For this review, use the dimensioned drawing (mm, ordinates from the lowest corner) and the shaded views. A direction names the side the tool comes from. Give positions to 0.01 mm unless a question says otherwise; leave off trailing zeros. Order: outer loops, then holes, each group sorted by start corner. A loop starts at its lowest first (then second) coordinate and runs counter-clockwise, first axis right, second up. Notation, with made-up numbers: M 57,-3 L 93,-3 A24 cw 93,26 Z; hole C 79.25,-17.5 d11. An arc over 180 degrees is marked long. Answer as CSV lines item,"result". Start each with the question number.
1. We need section A-A, the plane x = 6. Give the boundary of the cut face in (y, z), and give its area (3 significant figures).
2. We need section C-C, the plane z = 6. Give the boundary of the cut face in (x, y), and give its area (3 significant figures).
3. We need section B-B, the plane y = 3. Give the boundary of the cut face in (x, z), and give its area (3 significant figures).
4. We need section D-D, the plane y = 17.25. Give the boundary of the cut face in (x, z), and give its area (3 significant figures).
5. Clearance check with a flat-ended pin moving along its axis: P1, Ø5, axis at y = 18, z = 4.5, coming from the +X side. State where the tip first meets the part, or that it passes through.
6. For line 1 along X through (y, z) = (6, 6); line 2 along Y through (x, z) = (7.5, 3.5); line 3 along Y through (x, z) = (1.75, 3.5), list the stretches that pass through material, from the lowest coordinate up.
7. Mouldability with a two-part tool opening along X and no side actions: class the marked faces 3, 4 and 5 as pulls with the +X half, pulls with the -X half, needs draft (parallel to the pull), parting line crosses it, or undercut.
8. Machinability: for the marked faces 1 and 2, which of the approach directions +Z, -Z, +X, -X, +Y, -Y give a long, thin tool a straight path to every point of the face, cutting with its end or side? Answer none if there is none.
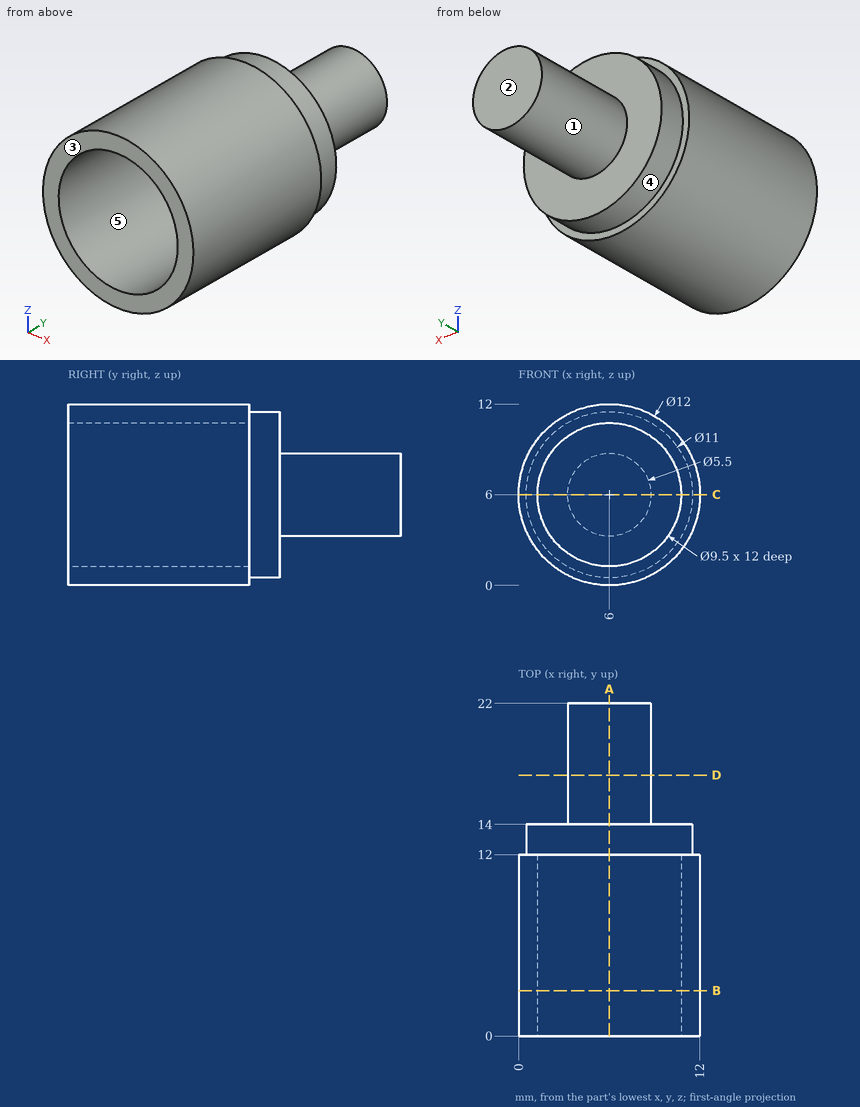
Result set:
1,outline,"M 0,0 L 12,0 L 12,0.5 L 14,0.5 L 14,3.25 L 22,3.25 L 22,8.75 L 14,8.75 L 14,11.5 L 12,11.5 L 12,12 L 0,12 L 0,10.75 L 12,10.75 L 12,1.25 L 0,1.25 Z"
1,area,"96.0 mm2"
2,outline,"M 0,0 L 1.25,0 L 1.25,12 L 10.75,12 L 10.75,0 L 12,0 L 12,12 L 11.5,12 L 11.5,14 L 8.75,14 L 8.75,22 L 3.25,22 L 3.25,14 L 0.5,14 L 0.5,12 L 0,12 Z"
2,area,"96.0 mm2"
3,outline,"C 6,6 d12; hole C 6,6 d9.5"
3,area,"42.2 mm2"
4,outline,"C 6,6 d5.5"
4,area,"23.8 mm2"
5,P1,"x = 8.75"
6,line 1,"0 to 1.25, 10.75 to 12"
6,line 2,"12 to 14"
6,line 3,"0 to 14"
7,face 3,"needs draft"
7,face 4,"parting line crosses it"
7,face 5,"undercut"
8,face 1,"+Y"
8,face 2,"+Z, -Z, +X, -X, +Y"
